Design review of the part shown in the three views and the two pictorial views. Dimensions are in mm from the part's minimum x, y and z. A direction names the side the tool comes from. Coordinates: 2 decimals unless noted, no trailing zeros. Write each loop counter-clockwise with the first axis right and the second up, starting at its lowest first coordinate (ties: lowest second). Pieces come first, ordered by that corner, then holes. Notation, with made-up numbers: (-27.75, 62.5) - (18.25, 62.5) arc R17 cw to (18.25, 86.5) - close; hole circle Ø6 at (44, 78.5). An arc over 180 degrees is marked (long way). Write each question's results on one line, items separated by ' | '.
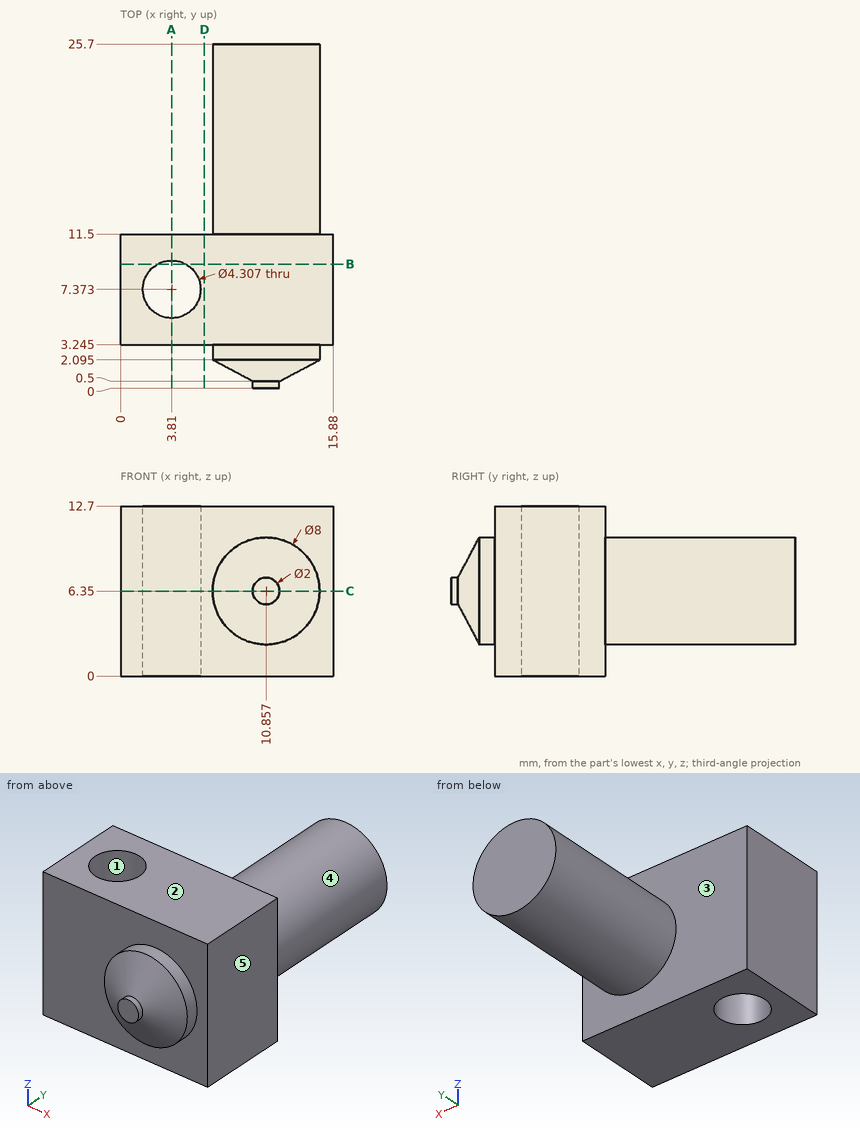
Q1. Mouldability with a two-part tool opening along Y and no side actions: class the marked faces 1, 2 and 3 as pulls with the +Y half, pulls with the -Y half, needs draft (parallel to the pull), parting line crosses it, or undercut.
Results found:
face 1: undercut | face 2: needs draft | face 3: pulls with the +Y half
Q2. Wall thickness on line 1 along Y through (x, z) = (3.81, 4.75) (1 decimal); line 2 along Y through (x, z) = (2.5, 5.75) (1 decimal); line 3 along Y through (x, z) = (6, 9) (1 decimal): over which ranges is each line inside the solid? List them lowest first. Write a range as from..to.
Results found:
line 1: 3.2..5.2, 9.5..11.5 | line 2: 3.2..5.7, 9.1..11.5 | line 3: 3.2..11.5
Q3. Take a section at D-D on x = 6.25. State the section outline as (y, z) points (1 decimal), plus the area to 3 significant figures.
Results found:
outline: (3.2, 0) - (11.5, 0) - (11.5, 12.7) - (3.2, 12.7) - close | area: 105 mm2
Q4. Take a section at B-B on y = 9.25. State the section outline as (x, z) points (1 decimal), plus the area to 3 significant figures.
Results found:
outline: (0, 0) - (2.8, 0) - (2.8, 12.7) - (0, 12.7) - close; (4.9, 0) - (15.9, 0) - (15.9, 12.7) - (4.9, 12.7) - close | area: 175 mm2
Q5. For pin 1 (4 mm diameter, centred on x = 5, z = 6.5, fed in from -Y); pin 2 (5 mm diameter, centred on x = 11.5, y = 5, fed in from -Z); pin 3 (5 mm diameter, centred on y = 20.5, z = 11, fed in from -X) (1 decimal); pin 4 (1 mm diameter, centred on x = 6.5, z = 4, fed in from +Y), all flat-tipped, find the tip position at first contact; note any pin that passes through.
Results found:
pin 1: y = 2.02 | pin 2: z = 0 | pin 3: x = 7.5 | pin 4: y = 11.5
Q6. Take a section at A-A on x = 3.81. State the section outline as (y, z) points (1 decimal).
Results found:
outline: (3.2, 0) - (5.2, 0) - (5.2, 12.7) - (3.2, 12.7) - close; (9.5, 0) - (11.5, 0) - (11.5, 12.7) - (9.5, 12.7) - close
Q7. Take a section at C-C on z = 6.35. State the section outline as (x, y) points (1 decimal).
Results found:
outline: (0, 3.2) - (6.9, 3.2) - (6.9, 2.1) - (9.9, 0.5) - (9.9, 0) - (11.9, 0) - (11.9, 0.5) - (14.9, 2.1) - (14.9, 3.2) - (15.9, 3.2) - (15.9, 11.5) - (14.9, 11.5) - (14.9, 25.7) - (6.9, 25.7) - (6.9, 11.5) - (0, 11.5) - close; hole circle Ø4.3 at (3.8, 7.4)
Q8. For the marked faces 4 and 5, list the 3-axis set-ups (+Z, -Z, +X, -X, +Y, -Y) from which the entire face can be reached by the end or side of a thin tool; tool diameter is ignored.
Results found:
face 4: +Y | face 5: +Z, -Z, +X, +Y, -Y
